from build123d import *

# Parameters (mm, degrees)
BOSS_EXTRUDE1_DEPTH = 3.175
CUT_EXTRUDE1_REACH  = 5.175
SKETCH2_W           = 29.718
SKETCH2_H           = 29.718
FILLET1_R           = 2.54
FILLET2_R           = 12.7


with BuildPart() as part:
    # Sketch1 → Boss-Extrude1 (new body)
    with BuildSketch(Plane.XY):
        with BuildLine():
            Line((-114.3, 203.2), (114.3, 203.2))
            ThreePointArc((114.3, 203.2), (148.443103792, 104.429956961), (152.4, 0))
            Line((152.4, 0), (158.711897248, -0.694588462))
            ThreePointArc((158.711897248, -0.694588462), (154.323359707, 107.497469491), (118.128585461, 209.55))
            ThreePointArc((118.128585461, 209.55), (0, 280.345753402), (-118.128585461, 209.55))
            ThreePointArc((-118.128585461, 209.55), (-154.323359707, 107.497469491), (-158.711897248, -0.694588462))
            Line((-158.711897248, -0.694588462), (-152.4, 0))
            ThreePointArc((-152.4, 0), (-148.443103792, 104.429956961), (-114.3, 203.2))
        make_face()
    extrude(amount=BOSS_EXTRUDE1_DEPTH)

    # Sketch2 → Cut-Extrude1 (cut, up to next)
    with BuildSketch(Plane.XY.offset(3.175), mode=Mode.PRIVATE) as cut_extrude1_sk1:
        with Locations((0, 241.772876701)):
            Rectangle(SKETCH2_W, SKETCH2_H)
    cut_extrude1_tool1 = extrude(cut_extrude1_sk1.sketch, amount=-CUT_EXTRUDE1_REACH, mode=Mode.PRIVATE) & part.part
    add(cut_extrude1_tool1.solids().sort_by_distance((0, 241.772877, 3.175))[0], mode=Mode.SUBTRACT)

    # Fillet1
    fillet1_edges = [part.edges().sort_by_distance(p)[0] for p in [
        (14.859, 256.631876701, 1.5875),
        (14.859, 226.913876701, 1.5875),
        (-14.859, 226.913876701, 1.5875),
        (-14.859, 256.631876701, 1.5875),
    ]]
    fillet(fillet1_edges, radius=FILLET1_R)

    # Fillet2
    fillet2_edges = [part.edges().sort_by_distance(p)[0] for p in [
        (-114.3, 203.2, 1.5875),
        (114.3, 203.2, 1.5875),
    ]]
    fillet(fillet2_edges, radius=FILLET2_R)


solid = part.part
The model under review builds one solid part; all positions refer to its coordinate system, in mm. A direction names the side the tool comes from. Round coordinates to 2 decimals unless told otherwise and drop trailing zeros. Loops run counter-clockwise (first coordinate to the right, second up) from the corner with the lowest first, then second, coordinate; pieces in that order, holes last. Notation, with made-up numbers: (-28, 18) -> (-24, 18) arc R8 ccw to (-24, 31) -> close; hole circle Ø1 at (25, 84). An arc over 180 degrees is marked (long way). One line per question, with ' | ' between items. Start each with the question number.
Item 1: Machinability: for faces 5 (the face through (154.61, 106, 1.57)), 6 (the face through (-149.4, 99.1, 1.6)), which of the approach directions +Z, -Z, +X, -X, +Y, -Y give a long, thin tool a straight path to every point of the face, cutting with its end or side? Answer none if there is none.
Item 2: Draft analysis for pull direction X (two halves, no side actions). For faces 1 (the face through (113.12, 201.34, 1.61)), 2 (the face through (-113.12, 201.34, 1.61)), 3 (the face through (2.02, 280.33, 1.57)), 4 (the face through (-1, 213, 0)), state which applies: +X half, -X half, draft (parallel to the pull), parting line (faces both ways), or undercut.
Item 3: Add section A-A, the plane z = 2.55. Write out the cut boundary in (x, y).
Item 4: Add section B-B, the plane y = 45. Write out the cut boundary in (x, z) (3 decimals), then the cut area to 3 significant figures.
Item 5: For pin 1 (1.6 mm diameter, centred on x = 46.5, z = 2, fed in from -Y); pin 2 (1 mm diameter, centred on y = 237, z = 2.5, fed in from +X), all flat-tipped, find the tip position at first contact; note any pin that passes through.
Item 6: Add section D-D, the plane x = 96. Write out the cut boundary in (y, z) (3 decimals), then the cut area to 3 significant figures.
Item 7: Wall thickness on line 1 along X through (y, z) = (33, 1.55); line 2 along Y through (x, z) = (-4, 0.3); line 3 along X through (y, z) = (231, 1.9): over which ranges is each line inside the solid? List them lowest first. Write a range as [from, to].
Item 8: Add section C-C, the plane x = -3. Write out the cut boundary in (y, z) (3 decimals).
Return value:
1) face 5: +Z, -Z, +X | face 6: +Z, -Z
2) face 1: undercut | face 2: undercut | face 3: parting line | face 4: draft
3) outline: (-158.71, -0.69) -> (-152.4, 0) arc R355.6 cw to (-117.89, 196.11) arc R12.7 cw to (-106.5, 203.2) -> (106.5, 203.2) arc R12.7 cw to (117.89, 196.11) arc R355.6 cw to (152.4, 0) -> (158.71, -0.69) arc R361.95 ccw to (118.13, 209.55) arc R133.95 ccw to (-118.13, 209.55) arc R361.95 ccw to start; hole (-14.86, 229.45) arc R2.54 ccw to (-12.32, 226.91) -> (12.32, 226.91) arc R2.54 ccw to (14.86, 229.45) -> (14.86, 254.09) arc R2.54 ccw to (12.32, 256.63) -> (-12.32, 256.63) arc R2.54 ccw to (-14.86, 254.09) -> close
4) outline: (-160.832, 0) -> (-154.481, 0) -> (-154.481, 3.175) -> (-160.832, 3.175) -> close; (154.481, 0) -> (160.832, 0) -> (160.832, 3.175) -> (154.481, 3.175) -> close | area: 40.3 mm2
5) pin 1: stops at y = 203.2 | pin 2: stops at x = 99.12
6) outline: (203.2, 0) -> (239.813, 0) -> (239.813, 3.175) -> (203.2, 3.175) -> close | area: 116 mm2
7) line 1: x = [-160.84, -154.48], [154.48, 160.84] | line 2: y = [203.2, 226.91], [256.63, 280.29] | line 3: x = [-103.85, -14.86], [14.86, 103.85]
8) outline: (203.2, 0) -> (226.914, 0) -> (226.914, 3.175) -> (203.2, 3.175) -> close; (256.632, 0) -> (280.312, 0) -> (280.312, 3.175) -> (256.632, 3.175) -> close
